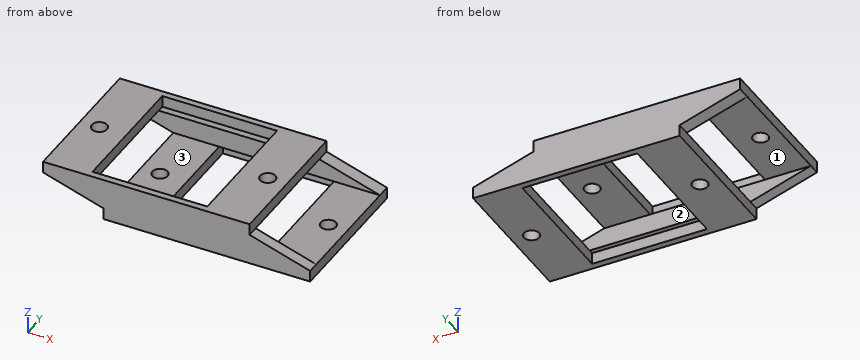
from build123d import *

# Parameters (mm, degrees)
SKETCH_1_W          = 54
SKETCH_1_H          = 38
EXTRUDE_1_DEPTH     = 3
SKETCH_3_R          = 2
SKETCH_3_W          = 30
SKETCH_3_H          = 34.54
CUT_EXTRUDE_1_DEPTH = 34.54
SKETCH_4_W          = 54
SKETCH_4_H          = 38
SKETCH_4_R          = 2
SKETCH_4_W_2        = 30
SKETCH_4_H_2        = 34.54
EXTRUDE_2_DEPTH     = 3
EXTRUDE_3_DEPTH     = 3.5
EXTRUDE_4_DEPTH     = 3


with BuildPart() as part:
    # Sketch 1 → Extrude 1 (new body)
    with BuildSketch(Plane.XY):
        with Locations((-8.445035234, 9.066128075)):
            Rectangle(SKETCH_1_W, SKETCH_1_H)
    extrude(amount=EXTRUDE_1_DEPTH)

    # Sketch 3 → Cut-Extrude 1 (cut)
    with BuildSketch(Plane(origin=(0, 0, 0), x_dir=(-1, 0, 0), z_dir=(0, 0, -1))):
        with Locations((-13.554964766, 8.526128075)):
            Circle(SKETCH_3_R)
        with Locations((30.445035234, 8.526128075)):
            Circle(SKETCH_3_R)
        with Locations((8.445035234, 9.092740444)):
            Rectangle(SKETCH_3_W, SKETCH_3_H)
    extrude(amount=-CUT_EXTRUDE_1_DEPTH, mode=Mode.SUBTRACT)



with BuildPart() as body_2:
    # Sketch 4 → Extrude 2 (new body)
    with BuildSketch(Plane(origin=(15.82462623, 0, -5), x_dir=(-1, 0, 0), z_dir=(0, 0, -1))):
        with Locations((8.445035234, 9.066128075)):
            Rectangle(SKETCH_4_W, SKETCH_4_H)
        with Locations((-13.554964766, 8.526128075)):
            Circle(SKETCH_4_R, mode=Mode.SUBTRACT)
        with Locations((30.445035234, 8.526128075)):
            Circle(SKETCH_4_R, mode=Mode.SUBTRACT)
        with Locations((8.445035234, 9.092740444)):
            Rectangle(SKETCH_4_W_2, SKETCH_4_H_2, mode=Mode.SUBTRACT)
    extrude(amount=EXTRUDE_2_DEPTH)


with BuildPart() as part_1:
    add(part.part)

    add(body_2.part)  # Extrude 3 merges body 2
    # Sketch 5 → Extrude 3 (add)
    with BuildSketch(Plane(origin=(0, 28.066128075, 0), x_dir=(1, 0, 0), z_dir=(0, 1, 0))):
        Polygon((-19.620409004, 5), (-35.445035234, 0), (18.554964766, 0), (34.379590996, 5), align=None)
    extrude(amount=-EXTRUDE_3_DEPTH)

    # Sketch 6 → Extrude 4 (add)
    with BuildSketch(Plane.XZ.offset(9.933871925)):
        Polygon((-35.445035234, 0), (-19.620409004, -5), (34.379590996, -5), (18.554964766, 0), align=None)
    extrude(amount=-EXTRUDE_4_DEPTH)


solid = part_1.part
The listing builds one solid part. Answer for the finished solid, in the listing's coordinates (mm). Face numbers are marked on the shaded views. A direction names the side the tool comes from. Give positions to 0.01 mm unless a question says otherwise; leave off trailing zeros. Order: outer loops, then holes, each group sorted by start corner. A loop starts at its lowest first (then second) coordinate and runs counter-clockwise, first axis right, second up. Notation, with made-up numbers: (60.5, 9.5) -> (104.5, 9.5) arc R9 cw to (104.5, 22.5) -> close; hole circle Ø6 at (-5.5, 57). An arc over 180 degrees is marked (long way). Put each result on its own line as item: value.
Item 1: Straight lines are drawn through the part: line 1 (X direction, y = -4, z = 2.25); line 2 (X direction, y = 23, z = -6.75); line 3 (Y direction, x = 17, z = -5.5). For each, find the intervals that lie inside material, in ascending order.
Established:
line 1: x = -35.45 to -23.45, 6.55 to 18.55
line 2: x = -19.62 to -7.62, 22.38 to 34.38
line 3: y = -9.93 to -8.18, 26.36 to 28.07
Item 2: For the marked faces 1, 2 and 3, determine the directions among +Z, -Z, +X, -X, +Y, -Y from which every point of the face is accessible in a straight line to the end or side of a thin tool.
Established:
face 1: -Z, +X, -X
face 2: +X, -X
face 3: +Z, +X, -X
Item 3: A cutting plane is placed at B-B on x = -2. Give the vertices of the cut face in (y, z).
Established:
outline: (-9.93, -8) -> (-8.18, -8) -> (-8.18, -5) -> (-6.93, -5) -> (-6.93, 0) -> (-8.18, 0) -> (-8.18, 3) -> (-9.93, 3) -> close; (24.57, -5) -> (26.36, -5) -> (26.36, -8) -> (28.07, -8) -> (28.07, 3) -> (26.36, 3) -> (26.36, 0) -> (24.57, 0) -> close
Item 4: A cutting plane is placed at A-A on y = -3. Give the vertices of the cut face in (x, z).
Established:
outline: (-35.45, 0) -> (-23.45, 0) -> (-23.45, 3) -> (-35.45, 3) -> close; (-19.62, -8) -> (-7.62, -8) -> (-7.62, -5) -> (-19.62, -5) -> close; (6.55, 0) -> (18.55, 0) -> (18.55, 3) -> (6.55, 3) -> close; (22.38, -8) -> (34.38, -8) -> (34.38, -5) -> (22.38, -5) -> close
Item 5: A cutting plane is placed at C-C on z = -0.75. Give the vertices of the cut face in (x, y), plus the area to 3 significant figures.
Established:
outline: (-33.07, -9.93) -> (20.93, -9.93) -> (20.93, -6.93) -> (-33.07, -6.93) -> close; (-33.07, 24.57) -> (20.93, 24.57) -> (20.93, 28.07) -> (-33.07, 28.07) -> close
area: 351 mm^2
Item 6: Given P1, Ø8, axis at x = -2.5, y = 4.5, coming from the +Z side; P2, Ø1.4, axis at x = -15.5, y = 25.5, coming from the +Z side; P3, Ø0.9, axis at y = 12.5, z = -7, coming from the -X side; P4, Ø2, axis at x = 18, y = 4, coming from the -Z side, each flat-ended and moving along its own axis, determine where each tip first touches the part or whether it passes through.
Established:
P1: passes through
P2: stops at z = 0
P3: stops at x = -19.62
P4: stops at z = 0
Item 7: A cutting plane is placed at D-D on x = 17. Give the vertices of the cut face in (y, z), plus the area to 3 significant figures.
Established:
outline: (-9.93, -8) -> (-8.18, -8) -> (-8.18, -5) -> (-6.93, -5) -> (-6.93, 0) -> (24.57, 0) -> (24.57, -5) -> (26.36, -5) -> (26.36, -8) -> (28.07, -8) -> (28.07, 3) -> (-9.93, 3) -> close
area: 157 mm^2
